Read the model definition and answer for the solid it produces. Units are mm, in the model's axes. Coordinates: 2 decimals unless noted, no trailing zeros. Loops run counter-clockwise (first coordinate to the right, second up) from the corner with the lowest first, then second, coordinate; pieces in that order, holes last.
Q1. Section D-D (z = -18) is taken. Give the vertices of the cut face in (x, y), then the cut area to 3 significant figures.
Q2. Section B-B (x = 0.9) is taken. Give the vertices of the cut face in (y, z) (3 decimals), then the cut area to 3 significant figures.
Q3. Straight lines are drawn through the part: line 1 (Y direction, x = 1.4, z = -19.5); line 2 (Z direction, x = 0.25, y = 62); line 3 (Z direction, x = 2.2, y = 114). For each, find the intervals that lie inside material, in ascending order.
Q4. Section C-C (y = 84) is taken. Give the vertices of the cut face in (x, z).
Q5. Section A-A (y = 126) is taken. Give the vertices of the cut face in (x, z), then the cut area to 3 significant figures.
Q6. Flat-ended cylindrical pins translate along their axes: P1, Ø0.9, axis at x = 1, y = -2, coming from the +Z side; P2, Ø1.5, axis at x = 1.5, y = -1, coming from the -Z side; P3, Ø1.5, axis at x = 1.5, z = 12.5, coming from the +Y side. Find the tip coordinate at first contact, or state that the pin passes through.
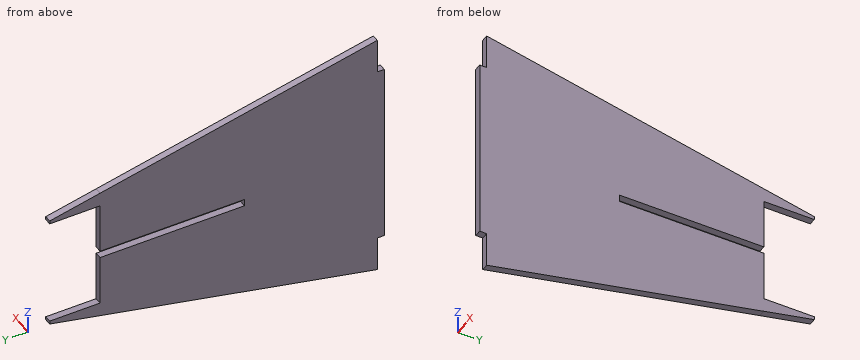
from build123d import *

# Parameters (mm, degrees)
EXTRUDE_1_DEPTH     = 3
BOSS_EXTRUDE1_DEPTH = 3


with BuildPart() as part:
    # Эскиз1 → Бобышка-Вытянуть1 (new body)
    with BuildSketch(Plane(origin=(0, 0, 0), x_dir=(0, 0, -1), z_dir=(1, 0, 0))):
        Polygon((29.113333333, 119), (54.5, 0), (39.5, 0), (39.5, -3), (-39.5, -3), (-39.5, 0), (-54.5, 0), (-29.113333333, 119), (-1.5, 119), (-1.5, 57), (1.5, 57), (1.5, 119), align=None)
    extrude(amount=EXTRUDE_1_DEPTH)

    # Sketch1 → Boss-Extrude1 (add)
    with BuildSketch(Plane(origin=(3, 0, 0), x_dir=(0, 0, -1), z_dir=(1, 0, 0))):
        Polygon((-29.113333333, 119), (-24.5, 140.625), (-23.113333333, 140.625), (-23.113333333, 119), align=None)
        Polygon((29.113333333, 119), (24.5, 140.625), (23.113333333, 140.625), (23.113333333, 119), align=None)
    extrude(amount=-BOSS_EXTRUDE1_DEPTH)


solid = part.part
Numbers:
1. outline: (0, -3) - (3, -3) - (3, 119) - (0, 119) - close
1. area: 366 mm2
2. outline: (-3, -39.5) - (0, -39.5) - (0, -54.5) - (140.625, -24.5) - (140.625, -23.113) - (119, -23.113) - (119, -1.5) - (57, -1.5) - (57, 1.5) - (119, 1.5) - (119, 23.113) - (140.625, 23.113) - (140.625, 24.5) - (0, 54.5) - (0, 39.5) - (-3, 39.5) - close
2. area: 10,200 mm2
3. line 1: y = -3 to 119
3. line 2: z = -41.27 to -1.5, 1.5 to 41.27
3. line 3: z = -30.18 to -1.5, 1.5 to 30.18
4. outline: (0, -36.58) - (3, -36.58) - (3, -1.5) - (0, -1.5) - close; (0, 1.5) - (3, 1.5) - (3, 36.58) - (0, 36.58) - close
5. outline: (0, -27.62) - (3, -27.62) - (3, -23.11) - (0, -23.11) - close; (0, 23.11) - (3, 23.11) - (3, 27.62) - (0, 27.62) - close
5. area: 27.0 mm2
6. P1: stops at z = 39.5
6. P2: stops at z = -39.5
6. P3: stops at y = 119
